Input: part model. Units: mm. Frame: model coordinates. Coordinates: 2 decimals unless noted, no trailing zeros. Loops run counter-clockwise (first coordinate to the right, second up) from the corner with the lowest first, then second, coordinate; pieces in that order, holes last. Notation, with made-up numbers: (10, 46.25) -> (19, 46.25) arc R21 ccw to (19, 51.25) -> close; hole circle Ø10 at (-6.5, 85.25). An arc over 180 degrees is marked (long way). Answer as a JSON object with one key per item and string values.
from build123d import *

# Parameters (mm, degrees)
SKETCH1_R           = 3
BOSS_EXTRUDE1_DEPTH = 50
CUT_EXTRUDE1_START  = -27.65
SKETCH2_R           = 3
CUT_EXTRUDE1_DEPTH  = 27.65
CUT_EXTRUDE2_START  = -20.15
SKETCH3_R           = 3
CUT_EXTRUDE2_DEPTH  = 20.15


with BuildPart() as part:
    # Sketch1 → Boss-Extrude1 (new, symmetric)
    with BuildSketch(Plane.XY):
        Circle(SKETCH1_R)
    extrude(amount=BOSS_EXTRUDE1_DEPTH, both=True)

    # Sketch2 → Cut-Extrude1 (cut)
    with BuildSketch(Plane.XY.offset(50).offset(CUT_EXTRUDE1_START)):
        Circle(SKETCH2_R)
    extrude(amount=CUT_EXTRUDE1_DEPTH, mode=Mode.SUBTRACT)

    # Sketch3 → Cut-Extrude2 (cut)
    with BuildSketch(Plane(origin=(0, 0, -50), x_dir=(-1, 0, 0), z_dir=(0, 0, -1)).offset(CUT_EXTRUDE2_START)):
        Circle(SKETCH3_R)
    extrude(amount=CUT_EXTRUDE2_DEPTH, mode=Mode.SUBTRACT)


solid = part.part
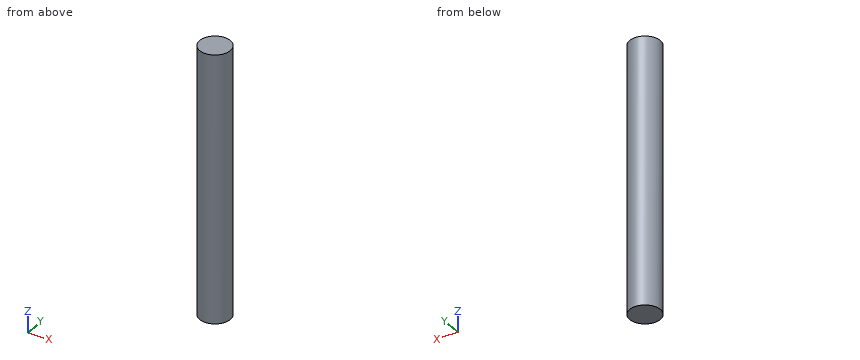
1. Line query: line 1 along Y through (x, z) = (1.35, -8); line 2 along X through (y, z) = (-2.75, 0); line 3 along Y through (x, z) = (0.15, -21). Output: solid intervals per line, ascending.
Reply:
{"line 1": "y = -2.68 to 2.68", "line 2": "x = -1.2 to 1.2", "line 3": "y = -3 to 3"}
2. Section query C-C (y = -0.85). Return loops of the section in (x, z), plus the area to 3 significant figures.
Reply:
{"outline": "(-2.88, -29.85) -> (2.88, -29.85) -> (2.88, 22.35) -> (-2.88, 22.35) -> close", "area": "300 mm2"}
3. Section query A-A (x = -1.8). Return loops of the section in (y, z).
Reply:
{"outline": "(-2.4, -29.85) -> (2.4, -29.85) -> (2.4, 22.35) -> (-2.4, 22.35) -> close"}
4. Pin query (flat end, axial travel): P1, Ø1, axis at y = -2.5, z = -22.5, coming from the +X side; P2, Ø1, axis at x = -1, z = -14, coming from the -Y side; P3, Ø1.5, axis at x = 1.5, z = 16, coming from the -Y side. Return the tip coordinate at first contact, or that it passes through.
Reply:
{"P1": "stops at x = 2.24", "P2": "stops at y = -2.96", "P3": "stops at y = -2.9"}
5. Section query B-B (z = 12.5). Return loops of the section in (x, y).
Reply:
{"outline": "circle Ø6 at (0, 0)"}
